from build123d import *

# Parameters (mm, degrees)
SKETCH1_R           = 2
SKETCH1_R_2         = 1.25
BOSS_EXTRUDE1_DEPTH = 3.175


with BuildPart() as part:
    # Sketch1 → Boss-Extrude1 (new body)
    with BuildSketch(Plane(origin=(0, 0, 0), x_dir=(1, 0, 0), z_dir=(0, 1, 0))):
        Polygon((0, 0), (230, 0), (230, 10), (230, 20), (200, 20), (200, 36.6), (195, 36.6), (190, 36.6), (190, 20), (30, 20), (30, 70), (15, 70), (0, 70), align=None)
        with Locations(Location((15, 10, 0), (0, 0, 270))):
            Circle(SKETCH1_R, mode=Mode.SUBTRACT)
        with BuildLine():
            ThreePointArc((148, 10), (150, 12), (152, 10))
            ThreePointArc((152, 10), (150, 8), (148, 10))
        make_face(mode=Mode.SUBTRACT)
        with Locations(Location((7, 47, 0), (0, 0, 270))):
            Circle(SKETCH1_R, mode=Mode.SUBTRACT)
        with Locations(Location((23, 47, 0), (0, 0, 270))):
            Circle(SKETCH1_R, mode=Mode.SUBTRACT)
        with BuildLine():
            ThreePointArc((10.050252532, 59.949747468), (12.321215973, 61.467156728), (15, 62))
            ThreePointArc((15, 62), (17.678784027, 48.532843272), (10.050252532, 59.949747468))
        make_face(mode=Mode.SUBTRACT)
        with Locations(Location((7, 63, 0), (0, 0, 270))):
            Circle(SKETCH1_R, mode=Mode.SUBTRACT)
        with Locations(Location((23, 63, 0), (0, 0, 270))):
            Circle(SKETCH1_R, mode=Mode.SUBTRACT)
        with Locations(Location((195, 28.3, 0), (0, 0, 270))):
            Circle(SKETCH1_R_2, mode=Mode.SUBTRACT)
    extrude(amount=BOSS_EXTRUDE1_DEPTH)


solid = part.part
For this review, take the finished solid that the model builds, in its own axes (mm). Give positions to 0.01 mm unless a question says otherwise; leave off trailing zeros. Loops run counter-clockwise (first coordinate to the right, second up) from the corner with the lowest first, then second, coordinate; pieces in that order, holes last. Notation, with made-up numbers: M 11.25,73.25 L 40.25,73.25 A26 cw 40.25,90.25 Z; hole C 89.5,3 d1. An arc over 180 degrees is marked long. Answer as a JSON object with one key per item and string values. Group by question number.
Q1. Add section A-A on x = 150. Give the boundary of the cut face in (y, z) (3 decimals).
Q2. Insertion check: P1, Ø1, axis at x = 196, y = 1, coming from the -Z side; P2, Ø12.5, axis at x = 15, z = -55, coming from the -Y side; P3, Ø1.6, axis at x = 209.5, y = 1, coming from the -Z side. Each pin has a flat end and moves straight along its axis. Give the tip position at first contact, or say it passes through.
Q3. Add section C-C on z = -55. Give the boundary of the cut face in (x, y) (3 decimals).
Q4. Add section B-B on y = 2.05. Give the number of separate pieces and of enclosed holes in the cut face, and give its area (3 significant figures).
Q5. For probe 1 along X at (y, z) = (2.65, -22.5); probe 2 along X at (y, z) = (0.4, -8.5); probe 3 along X at (y, z) = (0.8, -63), list the stretches that pass through material, from the lowest coordinate up. Write a range as [from, to].
Q6. Mouldability with a two-part tool opening along Z and no side actions: class faces 1 (the flat face through (113, 3.175, -12)), 2 (the cylindrical face through (148, 2, -10)) as +Z half, -Z half, draft (parallel to the pull), parting line (faces both ways), or undercut.
Checked values:
{
 "1": {"outline": "M 0,-20 L 3.175,-20 L 3.175,-12 L 0,-12 Z; M 0,-8 L 3.175,-8 L 3.175,0 L 0,0 Z"},
 "2": {"P1": "z = -36.6", "P2": "through", "P3": "z = -20"},
 "3": {"outline": "M 0,0 L 8,0 L 8,3.175 L 0,3.175 Z; M 22,0 L 30,0 L 30,3.175 L 22,3.175 Z"},
 "4": {"separate pieces": "1", "enclosed holes": "8", "area": "6,030 mm²"},
 "5": {"probe 1": "[0, 30], [190, 200]", "probe 2": "[0, 13.68], [16.32, 148.68], [151.32, 230]", "probe 3": "[0, 5], [9, 21], [25, 30]"},
 "6": {"face 1": "draft", "face 2": "undercut"}
}
